Could you check a few things on this model? Use its own coordinates, in mm. A direction names the side the tool comes from. Coordinates: 2 decimals unless noted, no trailing zeros.
1) Thinking about a two-plate mould opening in Z: for faces 1 (the face through (4, 15, 0)), 2 (the face through (4, 0, -15)), 3 (the face through (4, 11, 0)), which applies, released by +Z, released by -Z, zero draft, split by the parting line, or undercut?
2) Will these pins go through, and if not, where does the flat tip stop? P1, Ø1.5, axis at x = -7.5, z = 6.5, coming from the +Y side; P2, Ø1.2, axis at x = 50.5, z = -10.5, coming from the +Y side.
3) For faces 4 (the face through (271, 7, 0)), 5 (the face through (4, 0, -11.75)), which set-ups out of +Z, -Z, +X, -X, +Y, -Y let a thin tool reach every point of the face, with its end or its side?
4) If I drill on line 1 along Y through (x, z) = (-236, -13.55); line 2 along Y through (x, z) = (-88, 9.25); line 3 along Z through (x, y) = (-251, -13.05), over which ranges is the centre line in solid material (lowest first)?
5) Imagine slicing it at A-A on x = -64. Give the number of separate pieces and of enclosed holes in the cut face, plus the area to 3 significant figures.
```python
from build123d import *

# Parameters (mm, degrees)
SKETCH_1_W             = 23.5
SKETCH_1_H             = 12
EXTRUDE_1_DEPTH        = 271
HOLE_WIZARD_M6_1_D     = 5
HOLE_WIZARD_M6_1_DEPTH = 19
HOLE_WIZARD_M6_1_TIP   = 1.502151548
HOLE_WIZARD_M6_2_D     = 5
HOLE_WIZARD_M6_2_DEPTH = 19
HOLE_WIZARD_M6_2_TIP   = 1.502151548
HOLE_WIZARD_M4_1_D     = 3.3
HOLE_WIZARD_M4_1_DEPTH = 11.5
HOLE_WIZARD_M4_1_TIP   = 0.991420021


with BuildPart() as part:
    # 草图1 → 凸台-拉伸1 (new, symmetric)
    with BuildSketch(Plane(origin=(0, 0, 0), x_dir=(0, 0, -1), z_dir=(1, 0, 0))):
        Polygon((-15, 15), (-11.5, 15), (-11.5, 13.5), (-11, 13.5), (-11, 12), (-9.5, 12), (-9.5, 15), (-8, 15), (-8, 12.5), (-5, 12.5), (-5, 15), (5, 15), (5, 12.5), (8, 12.5), (8, 15), (9.5, 15), (9.5, 12), (11, 12), (11, 13.5), (11.5, 13.5), (11.5, 15), (15, 15), (15, 8), (12.5, 8), (12.5, 5), (15, 5), (15, -5), (12.5, -5), (12.5, -8), (15, -8), (15, -15), (11.5, -15), (11.5, -13.5), (11, -13.5), (11, -12), (9.5, -12), (9.5, -15), (8, -15), (8, -12.5), (5, -12.5), (5, -15), (-5, -15), (-5, -12.5), (-8, -12.5), (-8, -15), (-9.5, -15), (-9.5, -12), (-11, -12), (-11, -13.5), (-11.5, -13.5), (-11.5, -15), (-15, -15), align=None)
        with BuildLine():
            Line((12, -10.5), (12, -8.5))
            ThreePointArc((12, -8.5), (11.853553391, -8.146446609), (11.5, -8))
            Line((11.5, -8), (-11.5, -8))
            ThreePointArc((-11.5, -8), (-11.853553391, -8.146446609), (-12, -8.5))
            Line((-12, -8.5), (-12, -10.5))
            ThreePointArc((-12, -10.5), (-11.853553391, -10.853553391), (-11.5, -11))
            Line((-11.5, -11), (11.5, -11))
            ThreePointArc((11.5, -11), (11.853553391, -10.853553391), (12, -10.5))
        make_face(mode=Mode.SUBTRACT)
        with BuildLine():
            Line((-11.5, 11), (11.5, 11))
            ThreePointArc((11.5, 11), (11.853553391, 10.853553391), (12, 10.5))
            Line((12, 10.5), (12, 8.5))
            ThreePointArc((12, 8.5), (11.853553391, 8.146446609), (11.5, 8))
            Line((11.5, 8), (-11.5, 8))
            ThreePointArc((-11.5, 8), (-11.853553391, 8.146446609), (-12, 8.5))
            Line((-12, 8.5), (-12, 10.5))
            ThreePointArc((-12, 10.5), (-11.853553391, 10.853553391), (-11.5, 11))
        make_face(mode=Mode.SUBTRACT)
        Rectangle(SKETCH_1_W, SKETCH_1_H, mode=Mode.SUBTRACT)
    extrude(amount=EXTRUDE_1_DEPTH, both=True)

    # M6 螺纹孔1
    with Locations(Plane(origin=(0, -15, 0), x_dir=(-1, 0, 0), z_dir=(0, -1, 0))):
        with Locations((-236, 0), (-251, 0), (251, 0), (236, 0)):
            Hole(HOLE_WIZARD_M6_1_D / 2, depth=HOLE_WIZARD_M6_1_DEPTH)
            with Locations((0, 0, -(HOLE_WIZARD_M6_1_DEPTH + HOLE_WIZARD_M6_1_TIP / 2))):  # 118° drill point
                Cone(0, HOLE_WIZARD_M6_1_D / 2, HOLE_WIZARD_M6_1_TIP, mode=Mode.SUBTRACT)

    # M6 螺纹孔2
    with Locations(Plane(origin=(0, 0, -15), x_dir=(-1, 0, 0), z_dir=(0, 0, -1))):
        with Locations((236, 0), (251, 0)):
            Hole(HOLE_WIZARD_M6_2_D / 2, depth=HOLE_WIZARD_M6_2_DEPTH)
            with Locations((0, 0, -(HOLE_WIZARD_M6_2_DEPTH + HOLE_WIZARD_M6_2_TIP / 2))):  # 118° drill point
                Cone(0, HOLE_WIZARD_M6_2_D / 2, HOLE_WIZARD_M6_2_TIP, mode=Mode.SUBTRACT)

    # M4 螺纹孔1
    with Locations(Plane(origin=(0, 0, -15), x_dir=(-1, 0, 0), z_dir=(0, 0, -1))):
        with Locations((-258, 0), (-60.5, 0), (-21.500000001, 0), (200.999999999, 0)):
            Hole(HOLE_WIZARD_M4_1_D / 2, depth=HOLE_WIZARD_M4_1_DEPTH)
            with Locations((0, 0, -(HOLE_WIZARD_M4_1_DEPTH + HOLE_WIZARD_M4_1_TIP / 2))):  # 118° drill point
                Cone(0, HOLE_WIZARD_M4_1_D / 2, HOLE_WIZARD_M4_1_TIP, mode=Mode.SUBTRACT)


solid = part.part
```
Filled in:
1. face 1: zero draft
1. face 2: released by -Z
1. face 3: undercut
2. P1: stops at y = 12.5
2. P2: stops at y = 13.5
3. face 4: +Z, -Z, +X, +Y, -Y
3. face 5: +X, -X
4. line 1: y = -15 to -8, -5 to -2.5, 2.5 to 5, 8 to 15
4. line 2: y = -15 to -11, -8 to -6, 6 to 8, 11 to 15
4. line 3: z = -15 to -11, -9.5 to -8, -5 to -2.5, 2.5 to 5, 8 to 9.5, 11 to 15
5. separate pieces: 1
5. enclosed holes: 3
5. area: 408 mm2
